Read the model definition and answer for the solid it produces. Units are mm, in the model's axes. A direction names the side the tool comes from. Coordinates: 2 decimals unless noted, no trailing zeros. Loops run counter-clockwise (first coordinate to the right, second up) from the corner with the lowest first, then second, coordinate; pieces in that order, holes last. Notation, with made-up numbers: (48.5, 77.5) - (52.5, 77.5) arc R17 ccw to (52.5, 91.5) - close; hole circle Ø3 at (47.5, 86.5). An arc over 180 degrees is marked (long way). Use one line per item in the form item = value. Start each with the question number.
1) A cutting plane is placed at B-B (y = 398). Give the vertices of the cut face in (x, z), and give its area (4 significant figures).
2) A cutting plane is placed at C-C (x = -520). Give the vertices of the cut face in (y, z), and give its area (3 significant figures).
3) Each of these flat-tipped pins is pushed along its axis until it touches: P1, Ø8, axis at x = -101.71, y = 330.49, coming from the +Z side; P2, Ø12.5, axis at x = -99.5, z = 277, coming from the +Y side. Where does it stop, or does it pass through?
4) Consider line 1 (Z direction, x = -147, y = 422.5). Determine where the line is inside the solid, lowest interval first.
5) The mould has two halves that part along Y. Classify faces 4 (the face through (-103, -19.493, 133)), 5 (the face through (-301, 705.507, 4)), 6 (the face through (-301, -44.493, 5)), 7 (the face through (-471, 336, 0)): released by +Y, released by -Y, zero draft, split by the parting line, or undercut.
6) Which of the six approach directions +Z, -Z, +X, -X, +Y, -Y give full straight-line access (tool end or side, diameter ignored) to faces 1 (the face through (-115.575, 329, 269)), 2 (the face through (-103.3, 335.4, 260)), 3 (the face through (-416.9, 318.3, 5.1))?
7) A cutting plane is placed at A-A (z = 213). Give the vertices of the cut face in (x, y).
from build123d import *

# Parameters (mm, degrees)
F0_W     = 750
F0_H     = 750
F1_DEPTH = 10
F2_W     = 25
F2_H     = 25
F3_DEPTH = 250
F4_W     = 25
F4_H     = 749.966674
F5_DEPTH = 25
F6_R     = 5
F7_DEPTH = 285.001
F8_R     = 12.5
F9_DEPTH = 25


with BuildPart() as f1:
    # F0 (on Top) → F1 (new body)
    with BuildSketch(Plane.XY):
        with Locations((-465.575071, 330.507226)):
            Rectangle(F0_W, F0_H)
    extrude(amount=F1_DEPTH)

    # F2 (on face) → F3 (join)
    with BuildSketch(Plane.XY.offset(10)):
        with Locations((-103.075071, -31.992774)):
            Rectangle(F2_W, F2_H)
        with Locations((-103.075071, 693.007226)):
            Rectangle(F2_W, F2_H)
    extrude(amount=F3_DEPTH)

    # F4 (on face) → F5 (join)
    with BuildSketch(Plane.XY.offset(260)):
        with Locations((-103.075071, 330.490563)):
            Rectangle(F4_W, F4_H)
    extrude(amount=F5_DEPTH)

    # F6 (on face) → F7 (cut, through all)
    with BuildSketch(Plane.XY.offset(285)):
        with Locations((-101.70645, 330.490563)):
            Circle(F6_R)
    extrude(amount=-F7_DEPTH, mode=Mode.SUBTRACT)

    # F8 (on face) → F9 (cut)
    with BuildSketch(Plane.XY.offset(10)):
        with Locations((-414.20645, 330.507226)):
            Circle(F8_R)
    extrude(amount=-F9_DEPTH, mode=Mode.SUBTRACT)


solid = f1.part
Found:
q1.outline = (-840.58, 0) - (-90.58, 0) - (-90.58, 10) - (-840.58, 10) - close; (-115.58, 260) - (-90.58, 260) - (-90.58, 285) - (-115.58, 285) - close
q1.area = 8,125 mm^2
q2.outline = (-44.49, 0) - (705.51, 0) - (705.51, 10) - (-44.49, 10) - close
q2.area = 7,500 mm^2
q3.P1 = through
q3.P2 = 705.47
q4.line_1 = 0 to 10
q5.face_4 = undercut
q5.face_5 = released by +Y
q5.face_6 = released by -Y
q5.face_7 = zero draft
q6.face_1 = +Z, -X, +Y, -Y
q6.face_2 = +X, -X
q6.face_3 = +Z, -Z
q7.outline = (-115.58, -44.49) - (-90.58, -44.49) - (-90.58, -19.49) - (-115.58, -19.49) - close; (-115.58, 680.51) - (-90.58, 680.51) - (-90.58, 705.51) - (-115.58, 705.51) - close
